Verification items for the finished model (mm, model axes). Face numbers are marked on the shaded views. A direction names the side the tool comes from. Round coordinates to 2 decimals unless told otherwise and drop trailing zeros. Loops run counter-clockwise (first coordinate to the right, second up) from the corner with the lowest first, then second, coordinate; pieces in that order, holes last.
from build123d import *

# Parameters (mm, degrees)
F0_W            = 23
F0_H            = 22
F1_DEPTH        = 13
F2_W            = 8.1
F2_H            = 22
F3_DEPTH        = 17
F5_DEPTH        = 30
F7_DEPTH        = 25
F9_DEPTH        = 45
F10_DEPTH       = 40
F12_D           = 3.3
F12_DEPTH       = 14.5
F12_CBORE_D     = 7
F12_CBORE_DEPTH = 4
F12_TIP         = 0.9914200214
F13_DEPTH       = 3.05
F15_D           = 3.3
F15_DEPTH       = 14.5
F15_CBORE_D     = 7
F15_CBORE_DEPTH = 4
F15_TIP         = 0.9914200214
F16_DEPTH       = 3.05


with BuildPart() as f1:
    # F0 (on Top) → F1 (new body)
    with BuildSketch(Plane.XY):
        Rectangle(F0_W, F0_H)
    extrude(amount=F1_DEPTH)

    # F2 (on face) → F3 (join)
    with BuildSketch(Plane.XY.offset(13)):
        with Locations((7.45, 0)):
            Rectangle(F2_W, F2_H)
    extrude(amount=F3_DEPTH)

    # F4 (on face) → F5 (cut)
    with BuildSketch(Plane.XZ.offset(11)):
        with BuildLine():
            ThreePointArc((-9.5, 6.5), (-4.5, 1.5), (0.5, 6.5))
            ThreePointArc((0.5, 6.5), (-4.5, 11.5), (-9.5, 6.5))
        make_face()
    extrude(amount=-F5_DEPTH, mode=Mode.SUBTRACT)

    # F6 (on face) → F7 (cut)
    with BuildSketch(Plane.YZ.offset(11.5)):
        with BuildLine():
            ThreePointArc((-3.4807406984, 21.5), (3.2501853916, 15.50481661), (9.5, 22))
            Line((9.5, 22), (3, 22))
            Line((3, 22), (3, 21.5))
            Line((3, 21.5), (-3.4807406984, 21.5))
        make_face()
        with BuildLine():
            Line((3, 22), (9.5, 22))
            ThreePointArc((9.5, 22), (3.2501853916, 28.49518339), (-3.4807406984, 22.5))
            Line((-3.4807406984, 22.5), (3, 22.5))
            Line((3, 22.5), (3, 22))
        make_face()
        with BuildLine():
            Line((3, 21.5), (3, 22))
            Line((3, 22), (-3.5, 22))
            ThreePointArc((-3.5, 22), (-3.49518339, 21.7498146084), (-3.4807406984, 21.5))
            Line((-3.4807406984, 21.5), (3, 21.5))
        make_face()
        with BuildLine():
            Line((-3.5, 22), (3, 22))
            Line((3, 22), (3, 22.5))
            Line((3, 22.5), (-3.4807406984, 22.5))
            ThreePointArc((-3.4807406984, 22.5), (-3.49518339, 22.2501853916), (-3.5, 22))
        make_face()
        with BuildLine():
            ThreePointArc((-3.5, 22), (-3.49518339, 22.2501853916), (-3.4807406984, 22.5))
            Line((-3.4807406984, 22.5), (-15.5890611932, 22.5))
            Line((-15.5890611932, 22.5), (-15.5890611932, 22))
            Line((-15.5890611932, 22), (-3.5, 22))
        make_face()
        with BuildLine():
            Line((-15.5890611932, 21.5), (-3.4807406984, 21.5))
            ThreePointArc((-3.4807406984, 21.5), (-3.49518339, 21.7498146084), (-3.5, 22))
            Line((-3.5, 22), (-15.5890611932, 22))
            Line((-15.5890611932, 22), (-15.5890611932, 21.5))
        make_face()
    extrude(amount=-F7_DEPTH, mode=Mode.SUBTRACT)

    # F8 (on face) → F9 (cut)
    with BuildSketch(Plane.XZ.offset(11)):
        Polygon((27.05, 7), (-4.05, 7), (-4.05, 6.5), (-4.05, 6), (27.05, 6), align=None)
    extrude(amount=-F9_DEPTH, mode=Mode.SUBTRACT)

    # F6 (on face) → F10 (cut)
    with BuildSketch(Plane.YZ.offset(11.5)):
        with BuildLine():
            ThreePointArc((-3.4807406984, 21.5), (3.2501853916, 15.50481661), (9.5, 22))
            Line((9.5, 22), (3, 22))
            Line((3, 22), (3, 21.5))
            Line((3, 21.5), (-3.4807406984, 21.5))
        make_face()
        with BuildLine():
            Line((3, 22), (9.5, 22))
            ThreePointArc((9.5, 22), (3.2501853916, 28.49518339), (-3.4807406984, 22.5))
            Line((-3.4807406984, 22.5), (3, 22.5))
            Line((3, 22.5), (3, 22))
        make_face()
        with BuildLine():
            Line((3, 21.5), (3, 22))
            Line((3, 22), (-3.5, 22))
            ThreePointArc((-3.5, 22), (-3.49518339, 21.7498146084), (-3.4807406984, 21.5))
            Line((-3.4807406984, 21.5), (3, 21.5))
        make_face()
        with BuildLine():
            Line((-3.5, 22), (3, 22))
            Line((3, 22), (3, 22.5))
            Line((3, 22.5), (-3.4807406984, 22.5))
            ThreePointArc((-3.4807406984, 22.5), (-3.49518339, 22.2501853916), (-3.5, 22))
        make_face()
        with BuildLine():
            ThreePointArc((-3.5, 22), (-3.49518339, 22.2501853916), (-3.4807406984, 22.5))
            Line((-3.4807406984, 22.5), (-15.5890611932, 22.5))
            Line((-15.5890611932, 22.5), (-15.5890611932, 22))
            Line((-15.5890611932, 22), (-3.5, 22))
        make_face()
        with BuildLine():
            Line((-15.5890611932, 21.5), (-3.4807406984, 21.5))
            ThreePointArc((-3.4807406984, 21.5), (-3.49518339, 21.7498146084), (-3.5, 22))
            Line((-3.5, 22), (-15.5890611932, 22))
            Line((-15.5890611932, 22), (-15.5890611932, 21.5))
        make_face()
    extrude(amount=-F10_DEPTH, mode=Mode.SUBTRACT)

    # F12
    with Locations(Plane.XY.offset(30)):
        with Locations((7.45, -7)):
            CounterBoreHole(F12_D / 2, F12_CBORE_D / 2, F12_CBORE_DEPTH, depth=F12_DEPTH)
            with Locations((0, 0, -(F12_DEPTH + F12_TIP / 2))):  # 118° drill point
                Cone(0, F12_D / 2, F12_TIP, mode=Mode.SUBTRACT)

    # F11 (on face) → F13 (cut)
    with BuildSketch(Plane.XY.offset(30)):
        with BuildLine():
            ThreePointArc((7.45, -10.445), (9.8859828612, -9.4359828612), (10.895, -7))
            ThreePointArc((10.895, -7), (5.0140171388, -4.5640171388), (7.45, -10.445))
        make_face()
    extrude(amount=-F13_DEPTH, mode=Mode.SUBTRACT)

    # F15
    with Locations(Plane(origin=(0, 0, 0), x_dir=(1, 0, 0), z_dir=(0, 0, -1))):
        with Locations((7.5, 7), (7.5, -7)):
            CounterBoreHole(F15_D / 2, F15_CBORE_D / 2, F15_CBORE_DEPTH, depth=F15_DEPTH)
            with Locations((0, 0, -(F15_DEPTH + F15_TIP / 2))):  # 118° drill point
                Cone(0, F15_D / 2, F15_TIP, mode=Mode.SUBTRACT)

    # F14 (on face) → F16 (cut)
    with BuildSketch(Plane(origin=(0, 0, 0), x_dir=(1, 0, 0), z_dir=(0, 0, -1))):
        with BuildLine():
            ThreePointArc((7.5, 10.445), (5.0640171388, 4.5640171388), (10.945, 7))
            Line((10.945, 7), (7.5, 7))
            Line((7.5, 7), (7.5, 10.445))
        make_face()
        with BuildLine():
            Line((7.5, 7), (10.945, 7))
            ThreePointArc((10.945, 7), (9.9359828612, 9.4359828612), (7.5, 10.445))
            Line((7.5, 10.445), (7.5, 7))
        make_face()
        with BuildLine():
            ThreePointArc((10.945, -7), (5.0640171388, -4.5640171388), (7.5, -10.445))
            Line((7.5, -10.445), (7.5, -7))
            Line((7.5, -7), (10.945, -7))
        make_face()
        with BuildLine():
            Line((7.5, -7), (7.5, -10.445))
            ThreePointArc((7.5, -10.445), (9.9359828612, -9.4359828612), (10.945, -7))
            Line((10.945, -7), (7.5, -7))
        make_face()
    extrude(amount=-F16_DEPTH, mode=Mode.SUBTRACT)


solid = f1.part
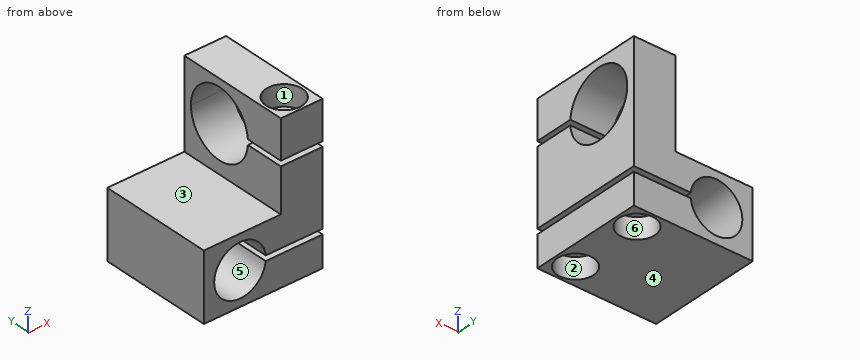
1. Section check A-A (z = 9.5). Enter the section's corners in (x, y).
2. Gauge pin test, flat ends, axial feed: P1, Ø3.5, axis at x = 9, y = 7, coming from the -Z side; P2, Ø6, axis at x = 0.5, z = 13.5, coming from the +Y side; P3, Ø4.5, axis at x = -4.5, y = 5.5, coming from the +Z side; P4, Ø4, axis at x = 7.5, y = -7, coming from the +Z side. Record the tip position at first contact, or that the pin passes through.
3. Section check D-D (y = 1.5). Enter the section's corners in (x, z), then the cut area to 3 significant figures.
4. Scan lines: L1, parallel to Y at x = 7.5, z = 13; L2, parallel to Y at x = 7.5, z = 1.45; L3, parallel to Z at x = -4.5, y = -9. Record each from-to range of solid material in increasing order.
5. Section check B-B (x = -4.5). Enter the section's corners in (y, z).
6. Section check C-C (z = 23). Enter the section's corners in (x, y).
7. Tool access check on the marked faces 1, 2 and 3. Record the directions out of +Z, -Z, +X, -X, +Y, -Y that give a thin tool (end or side, any length) a straight path to the whole face; none if there is none.
8. Release check for a two-part mould opening along Z. For the marked faces 4, 5 and 6 record: released by +Z, released by -Z, zero draft, split by the parting line, or undercut.
Taken from the geometry:
1. outline: (-11.5, -11) - (-8.5, -11) - (-8.5, 11) - (-11.5, 11) - close; (-0.5, -11) - (11.5, -11) - (11.5, 11) - (-0.5, 11) - close; hole circle Ø3.3 at (7.5, -7); hole circle Ø3.3 at (7.5, 7)
2. P1: stops at z = 4
2. P2: stops at y = 11
2. P3: stops at z = 13
2. P4: stops at z = 26
3. outline: (-11.5, 0) - (11.5, 0) - (11.5, 6) - (0.47, 6) arc R5 cw (long way) to (0.47, 7) - (11.5, 7) - (11.5, 15.68) - (3.4, 15.68) - (3.4, 13) - (-11.5, 13) - close; (3.4, 28.32) - (11.5, 28.32) - (11.5, 30) - (3.4, 30) - close
3. area: 245 mm2
4. L1: y = -11 to -8.65, -5.35 to 5.35, 8.65 to 11
4. L2: y = -11 to -10.5, -3.5 to 3.5, 10.5 to 11
4. L3: z = 0 to 1.5, 11.5 to 13
5. outline: (-11, 0) - (11, 0) - (11, 1.5) - (-11, 1.5) - close; (-11, 11.5) - (11, 11.5) - (11, 13) - (-11, 13) - close
6. outline: (3.4, -11) - (11.5, -11) - (11.5, -3.42) - (3.4, -3.42) - close; (3.4, 9.42) - (11.5, 9.42) - (11.5, 11) - (3.4, 11) - close; hole circle Ø3.3 at (7.45, -7)
7. face 1: +Z
7. face 2: -Z
7. face 3: +Z, -X, +Y, -Y
8. face 4: released by -Z
8. face 5: undercut
8. face 6: zero draft
